from build123d import *

# Parameters (mm, degrees)
SKETCH1_R           = 10.16
SKETCH1_R_2         = 2
BOSS_EXTRUDE1_DEPTH = 12.7
SKETCH2_R           = 14.2875
CUT_EXTRUDE1_DEPTH  = 7.9375


with BuildPart() as part:
    # Sketch1 → Boss-Extrude1 (new body)
    with BuildSketch(Plane.XY):
        Polygon((14, -56), (-32, -56), (-32, 0), (-32, 30), (32, 30), (32, -28.77498914), (14, -28.77498914), align=None)
        Circle(SKETCH1_R, mode=Mode.SUBTRACT)
        with Locations((-19, -45.77498914)):
            Circle(SKETCH1_R_2, mode=Mode.SUBTRACT)
    extrude(amount=BOSS_EXTRUDE1_DEPTH)

    # Sketch2 → Cut-Extrude1 (cut)
    with BuildSketch(Plane.XY):
        Circle(SKETCH2_R)
    extrude(amount=CUT_EXTRUDE1_DEPTH, mode=Mode.SUBTRACT)


solid = part.part
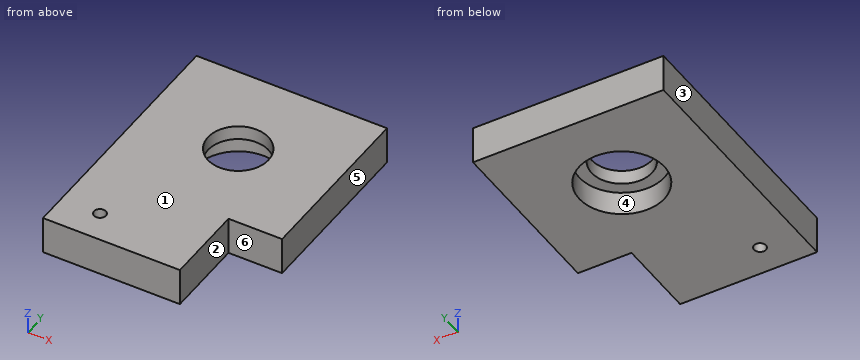
CAD build for the part. Positions are in the model's coordinates, mm. Face numbers are marked on the shaded views. A direction names the side the tool comes from. Round coordinates to 2 decimals unless told otherwise and drop trailing zeros. Loops run counter-clockwise (first coordinate to the right, second up) from the corner with the lowest first, then second, coordinate; pieces in that order, holes last.
(1) Wall check: line 1 along X through (y, z) = (0, 9); line 2 along Y through (x, z) = (-19, 3.75); line 3 along Y through (x, z) = (0, 3.75). Give the ranges that are in metal, low to high.
(2) Two-plate mould, pull along X, no slides. Class the marked faces 3, 4, 5 and 6: +X half, -X half, draft (parallel to the pull), parting line (faces both ways), or undercut.
(3) Cut at A-A (x = -19). Give the cut face in (y, z).
(4) Cut at B-B (y = 4). Give the cut face in (x, z).
(5) Cut at C-C (z = 9.5). Give the cut face in (x, y), plus the area to 3 significant figures.
(6) Cut at D-D (x = 8.5). Give the cut face in (y, z), plus the area to 3 significant figures.
(7) Which spindle directions (+Z, -Z, +X, -X, +Y, -Y) get a long thin tool onto all of the face, cutting with end or side? Do the marked faces 1 and 2. Say none if no direction does.
Findings below:
1. line 1: x = -32 to -10.16, 10.16 to 32
1. line 2: y = -56 to -47.77, -43.77 to 30
1. line 3: y = -56 to -14.29, 14.29 to 30
2. face 3: -X half
2. face 4: undercut
2. face 5: +X half
2. face 6: draft
3. outline: (-56, 0) - (-47.77, 0) - (-47.77, 12.7) - (-56, 12.7) - close; (-43.77, 0) - (30, 0) - (30, 12.7) - (-43.77, 12.7) - close
4. outline: (-32, 0) - (-13.72, 0) - (-13.72, 7.94) - (-9.34, 7.94) - (-9.34, 12.7) - (-32, 12.7) - close; (9.34, 7.94) - (13.72, 7.94) - (13.72, 0) - (32, 0) - (32, 12.7) - (9.34, 12.7) - close
5. outline: (-32, -56) - (14, -56) - (14, -28.77) - (32, -28.77) - (32, 30) - (-32, 30) - close; hole circle Ø4 at (-19, -45.77); hole circle Ø20.32 at (0, 0)
5. area: 4,680 mm2
6. outline: (-56, 0) - (-11.48, 0) - (-11.48, 7.94) - (-5.57, 7.94) - (-5.57, 12.7) - (-56, 12.7) - close; (5.57, 7.94) - (11.48, 7.94) - (11.48, 0) - (30, 0) - (30, 12.7) - (5.57, 12.7) - close
6. area: 857 mm2
7. face 1: +Z, +X, -X, +Y, -Y
7. face 2: +Z, -Z, +X, -Y
